Geometry: final body of the model. Coordinates: model frame, mm. A direction names the side the tool comes from. Give positions to 0.01 mm unless a question says otherwise; leave off trailing zeros. Order: outer loops, then holes, each group sorted by start corner. A loop starts at its lowest first (then second) coordinate and runs counter-clockwise, first axis right, second up. Notation, with made-up numbers: (12.5, 44.25) -> (29.5, 44.25) arc R17 ccw to (29.5, 66.25) -> close; hole circle Ø8 at (62.5, 71.25). An arc over 180 degrees is marked (long way). One line per item, written item: value. Start each with the question number.
Autodesk Inventor part; units mm, degrees
ref_plane "YZ Plane" through (0, 0, 0) normal (1, 0, 0) x (0, 1, 0)
ref_plane "XZ Plane" through (0, 0, 0) normal (0, 1, 0) x (-1, 0, 0)
ref_plane "XY Plane" through (0, 0, 0) normal (0, 0, 1) x (1, 0, 0)
sketch "Sketch1" plane through (0, 0, 0) normal (0, 0, 1) x (1, 0, 0)
  circle A0 centre (4, 4) radius 1.2
  circle A1 centre (4, 4) radius 1.5
  point P0 (0, 0)
  dimension "d0" = 3
extrude "Extrusion1" add sketch "Sketch1" against normal blind 8 contours A0 | A1
sketch "Sketch2" plane through (4, 4, 0) normal (0, 0, 1) x (1, 0, 0)
  circle A0 centre (0, 0) radius 1.5
  circle A1 centre (0, 0) radius 2.8
  point P0 (-4, -4)
  dimension "d3" = 5.6
extrude "Extrusion2" add sketch "Sketch2" along normal blind 3 contours A0 | A1
fillet "Fillet1" radius 0.3 1 edges at (1.2, 4, 3)
sketch "Sketch3" plane through (4, 4, 0) normal (0, 0, -1) x (-1, 0, 0)
  circle A0 centre (0, 0) radius 2.8
  circle A1 centre (0, 0) radius 1.5
  circle A2 centre (0, 0) radius 2.75
  point P0 (4, -4)
  dimension "d7" = 5.5
extrude "Extrusion3" cut sketch "Sketch3" against normal blind 0.5 contours A0
sketch "Sketch4" plane through (4, 4, 3) normal (0, 0, 1) x (1, 0, 0)
  circle A0 centre (0, 0) radius 2.5
  line L0 (0.7217, 1.25) -> (1.4434, 0)
  line L1 (1.4434, 0) -> (0.7217, -1.25)
  line L2 (0.7217, -1.25) -> (-0.7217, -1.25)
  line L3 (-0.7217, -1.25) -> (-1.4434, 0)
  line L4 (-1.4434, 0) -> (-0.7217, 1.25)
  line L5 (-0.7217, 1.25) -> (0.7217, 1.25)
  point P0 (-4, -4)
  dimension "d10" = 2.5
extrude "Extrusion4" cut sketch "Sketch4" against normal blind 2 contours L0 L1 L2 L3 L4 L5
thread "Thread1"
properties part number "m3 6" material "Steel"
1. Material intervals for L1, parallel to Z at x = 6.25, y = 3; L2, parallel to Y at x = 3.85, z = 2; L3, parallel to Z at x = 4.45, y = 2.95, sorted ascending. Write a range as [from, to].
2. Pin query (flat end, axial travel): P1, Ø3, axis at y = 2.5, z = -2.5, coming from the -X side; P2, Ø1, axis at y = 2.5, z = 1, coming from the +X side. Return the tip coordinate at first contact, or that it passes through.
3. Cut plane A-A, the plane z = 1.25. Return loops of the section in (x, y), then the cut area to 3 significant figures.
4. Draft query along Y for faces 4 (the cylindrical face through (2.73, 1.56, 0.25)), 5 (the flat face through (5.2, 2.8, 0)), 6 (the flat face through (2.92, 3.37, 2.01)). Return one class per face: pulls with the +Y half, pulls with the -Y half, needs draft (parallel to the pull), parting line crosses it, or undercut.
5. Cut plane B-B, the plane x = 4. Return loops of the section in (y, z), then the cut area to 3 significant figures.
6. Cut plane C-C, the plane z = -3. Return loops of the section in (x, y), then the cut area to 3 significant figures.
7. Access query for faces 1 (the flat face through (5.1, 2.9, 3)), 2 (the flat face through (4, 2.75, 2)), 3 (the cylindrical face through (5.43, 4.45, -3.94)). Directions: +Z, -Z, +X, -X, +Y, -Y. A direction counts if a zero-diameter tool reaches every point of the face in a straight line with its end or side. Return the directions, or none.
Answers follow:
1. L1: z = [0, 3]
1. L2: y = [1.2, 2.75], [5.25, 6.8]
1. L3: z = [-8, 1]
2. P1: stops at x = 2.5
2. P2: stops at x = 6.62
3. outline: circle Ø5.6 at (4, 4); hole (2.56, 4) -> (3.28, 2.75) -> (4.72, 2.75) -> (5.44, 4) -> (4.72, 5.25) -> (3.28, 5.25) -> close
3. area: 19.2 mm²
4. face 4: parting line crosses it
4. face 5: needs draft
4. face 6: undercut
5. outline: (1.2, 0.5) -> (1.25, 0.5) -> (1.25, 0) -> (2.5, 0) -> (2.5, -8) -> (5.5, -8) -> (5.5, 0) -> (6.75, 0) -> (6.75, 0.5) -> (6.8, 0.5) -> (6.8, 2.7) arc R0.3 ccw to (6.5, 3) -> (5.25, 3) -> (5.25, 1) -> (2.75, 1) -> (2.75, 3) -> (1.5, 3) arc R0.3 ccw to (1.2, 2.7) -> close
5. area: 35.7 mm²
6. outline: circle Ø3 at (4, 4)
6. area: 7.07 mm²
7. face 1: +Z, +X, -X, +Y, -Y
7. face 2: +Z
7. face 3: -Z
